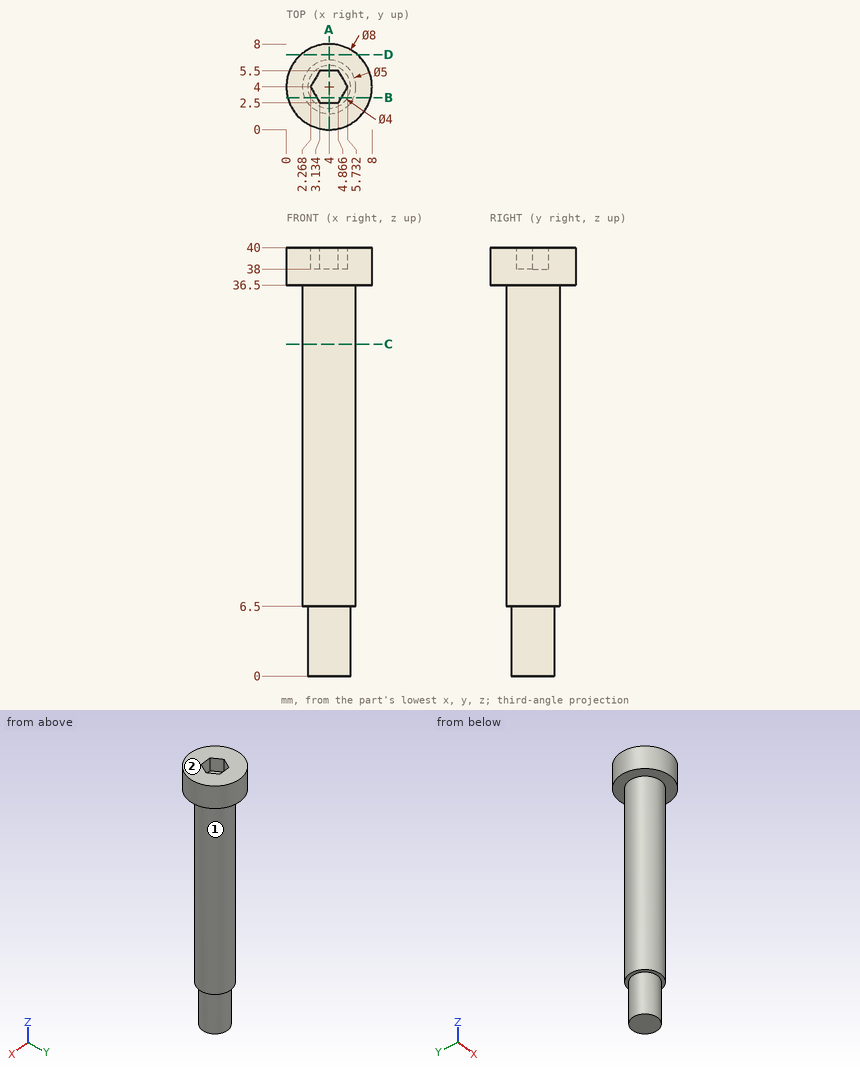
Check sheet for the drawn part. Datum: minimum x, y, z corner. Units: mm. A direction names the side the tool comes from. Coordinates: 2 decimals unless noted, no trailing zeros. Write each loop counter-clockwise with the first axis right and the second up, starting at its lowest first coordinate (ties: lowest second). Pieces come first, ordered by that corner, then holes. Notation, with made-up numbers: (68, -3) - (99, -3) arc R24 cw to (99, 28) - close; hole circle Ø8 at (-19.75, 54.25). An arc over 180 degrees is marked (long way). Answer as a JSON object with one key per item and string values.
(1) Cross-section at A-A on x = 4. Record the cut outline in (y, z).
Report:
{"outline": "(0, 36.5) - (1.5, 36.5) - (1.5, 6.5) - (2, 6.5) - (2, 0) - (6, 0) - (6, 6.5) - (6.5, 6.5) - (6.5, 36.5) - (8, 36.5) - (8, 40) - (5.5, 40) - (5.5, 38) - (2.5, 38) - (2.5, 40) - (0, 40) - close"}
(2) Gauge pin test, flat ends, axial feed: pin 1 Ø1.5 at (x, y) = (5, 3) entering from -Z; pin 2 Ø3 at (x, z) = (1, 35.5) entering from -Y; pin 3 Ø2 at (x, z) = (4, 11.5) entering from +Y. Record the tip position at first contact, or that the pin passes through.
Report:
{"pin 1": "z = 0", "pin 2": "y = 0.47", "pin 3": "y = 6.5"}
(3) Cross-section at C-C on z = 31. Record the cut outline in (x, y), plus the area to 3 significant figures.
Report:
{"outline": "circle Ø5 at (4, 4)", "area": "19.6 mm^2"}
(4) Cross-section at D-D on y = 7. Record the cut outline in (x, z).
Report:
{"outline": "(1.35, 36.5) - (6.65, 36.5) - (6.65, 40) - (1.35, 40) - close"}
(5) Tool access check on the marked faces 1 and 2. Record the directions out of +Z, -Z, +X, -X, +Y, -Y that give a thin tool (end or side, any length) a straight path to the whole face; none if there is none.
Report:
{"face 1": "-Z", "face 2": "+Z, +X, -X, +Y, -Y"}
(6) Cross-section at B-B on y = 3. Record the cut outline in (x, z).
Report:
{"outline": "(0.13, 36.5) - (1.71, 36.5) - (1.71, 6.5) - (2.27, 6.5) - (2.27, 0) - (5.73, 0) - (5.73, 6.5) - (6.29, 6.5) - (6.29, 36.5) - (7.87, 36.5) - (7.87, 40) - (5.15, 40) - (5.15, 38) - (2.85, 38) - (2.85, 40) - (0.13, 40) - close"}
(7) Thickness scan on line 1 along Z through (x, y) = (2.25, 2.75); line 2 along Y through (x, z) = (4, 21); line 3 along Y through (x, z) = (2.5, 25.5). Record the ranges inside material, lowest first.
Report:
{"line 1": "6.5 to 40", "line 2": "1.5 to 6.5", "line 3": "2 to 6"}
